Verification items for the finished model (mm, model axes). A direction names the side the tool comes from. Coordinates: 2 decimals unless noted, no trailing zeros. Write each loop counter-clockwise with the first axis right and the second up, starting at its lowest first coordinate (ties: lowest second). Pieces come first, ordered by that corner, then holes. Notation, with made-up numbers: M 73,45 L 108,45 A15 cw 108,58 Z; hole C 71.25,63 d11. An arc over 180 degrees is marked long. Answer in a Markdown table with one row per item.
from build123d import *

# Parameters (mm, degrees)
SKETCH1_W               = 80
SKETCH1_H               = 22
BOSS_EXTRUDE1_DEPTH     = 24
SKETCH2_R               = 3.85
EYESHAFT_HOLES_DEPTH    = 15
SKETCH5_W               = 5
SKETCH5_H               = 2.2
FRONT_LEG_HOLES_DEPTH   = 13
SKETCH6_W               = 20
SKETCH6_H               = 24
SERVO_BLOCK_DEPTH       = 17.5
SKETCH7_W               = 10.2
SKETCH7_H               = 3.3
BACK_LEGS_DEPTH         = 13
FILLET1_R               = 3
SKETCH8_R               = 2.714277304
CUT_EXTRUDE4_DEPTH      = 14
SKETCH9_W               = 12.2
SKETCH9_H               = 33.2
SERVO_ARMS1_DEPTH       = 11.6
FILLET2_R               = 2
CHAMFER1_SIZE           = 1
SKETCH14_W              = 12.4
SKETCH14_H              = 25
CUT_EXTRUDE5_DEPTH      = 11
SKETCH15_W              = 9
SKETCH15_H              = 4
CUT_EXTRUDE6_DEPTH      = 5.5
SKETCH16_W              = 5
SKETCH16_H              = 1
CUT_EXTRUDE7_DEPTH      = 11
SKETCH13_R              = 0.5
SERVO_SCREW_HOLES_DEPTH = 2
FILLET3_R               = 2


with BuildPart() as part:
    # Sketch1 → Boss-Extrude1 (new body)
    with BuildSketch(Plane(origin=(0, 0, 0), x_dir=(1, 0, 0), z_dir=(0, 1, 0))):
        Rectangle(SKETCH1_W, SKETCH1_H)
    extrude(amount=BOSS_EXTRUDE1_DEPTH)

    # Sketch2 → Eyeshaft holes (cut)
    with BuildSketch(Plane(origin=(0, 24, 0), x_dir=(1, 0, 0), z_dir=(0, 1, 0))):
        with Locations(Location((-30, -5, 0), (0, 0, 270))):
            Circle(SKETCH2_R)
        with Locations(Location((30, -5, 0), (0, 0, 270))):
            Circle(SKETCH2_R)
    extrude(amount=-EYESHAFT_HOLES_DEPTH, mode=Mode.SUBTRACT)

    # Sketch5 → Front leg holes (cut)
    with BuildSketch(Plane(origin=(0, 24, 0), x_dir=(1, 0, 0), z_dir=(0, 1, 0))):
        with Locations((-20, -5)):
            Rectangle(SKETCH5_W, SKETCH5_H)
        with Locations((20, -5)):
            Rectangle(SKETCH5_W, SKETCH5_H)
    extrude(amount=-FRONT_LEG_HOLES_DEPTH, mode=Mode.SUBTRACT)

    # Sketch6 → Servo block (add, symmetric)
    with BuildSketch(Plane.XY):
        with Locations((0, 12)):
            Rectangle(SKETCH6_W, SKETCH6_H)
    extrude(amount=SERVO_BLOCK_DEPTH, both=True)

    # Sketch7 → Back Legs (cut)
    with BuildSketch(Plane(origin=(0, 24, 0), x_dir=(1, 0, 0), z_dir=(0, 1, 0))):
        with Locations((-25.75, 3.4)):
            Rectangle(SKETCH7_W, SKETCH7_H)
        with Locations((25, 3.45)):
            Rectangle(SKETCH7_W, SKETCH7_H)
    extrude(amount=-BACK_LEGS_DEPTH, mode=Mode.SUBTRACT)

    # Fillet1
    fillet1_edges = [part.edges().sort_by_distance(p)[0] for p in [
        (-30, 9, 1.15),
        (30, 9, 1.15),
    ]]
    fillet(fillet1_edges, radius=FILLET1_R)

    # Sketch8 → Cut-Extrude4 (cut)
    with BuildSketch(Plane(origin=(0, 24, 0), x_dir=(1, 0, 0), z_dir=(0, 1, 0))):
        with Locations(Location((0, -5, 0), (0, 0, 270))):
            Circle(SKETCH8_R)
    extrude(amount=-CUT_EXTRUDE4_DEPTH, mode=Mode.SUBTRACT)

    # Sketch9 → Servo arms1 (cut)
    with BuildSketch(Plane(origin=(0, 24, 0), x_dir=(1, 0, 0), z_dir=(0, 1, 0))):
        Rectangle(SKETCH9_W, SKETCH9_H)
    extrude(amount=-SERVO_ARMS1_DEPTH, mode=Mode.SUBTRACT)

    # Fillet2
    fillet2_edges = [part.edges().sort_by_distance(p)[0] for p in [
        (10, 12, -11),
        (10, 12, -17.5),
        (10, 12, 11),
        (-10, 12, -11),
        (-10, 12, -17.5),
        (-10, 12, 11),
        (10, 12, 17.5),
        (-10, 12, 17.5),
        (40, 12, 11),
        (-40, 12, 11),
        (-40, 12, -11),
        (40, 12, -11),
    ]]
    fillet(fillet2_edges, radius=FILLET2_R)

    # Chamfer1
    chamfer1_edges = [part.edges().sort_by_distance(p)[0] for p in [
        (-30, 24, 1.15),
        (30, 24, 1.15),
        (-17.5, 24, 5),
        (-20, 24, 3.9),
        (-22.5, 24, 5),
        (-20, 24, 6.1),
        (22.5, 24, 5),
        (20, 24, 3.9),
        (17.5, 24, 5),
        (20, 24, 6.1),
        (-30.85, 24, -3.4),
        (-25.75, 24, -1.75),
        (-20.65, 24, -3.4),
        (-25.75, 24, -5.05),
        (19.9, 24, -3.45),
        (25, 24, -1.8),
        (30.1, 24, -3.45),
        (25, 24, -5.1),
    ]]
    chamfer(chamfer1_edges, length=CHAMFER1_SIZE)

    # Sketch14 → Cut-Extrude5 (cut)
    with BuildSketch(Plane(origin=(0, 12.4, 0), x_dir=(1, 0, 0), z_dir=(0, 1, 0))):
        with Locations((0, 0.5)):
            Rectangle(SKETCH14_W, SKETCH14_H)
    extrude(amount=-CUT_EXTRUDE5_DEPTH, mode=Mode.SUBTRACT)

    # Sketch15 → Cut-Extrude6 (cut)
    with BuildSketch(Plane.XY.offset(17.5)):
        with Locations((0, 3.4)):
            Rectangle(SKETCH15_W, SKETCH15_H)
    extrude(amount=-CUT_EXTRUDE6_DEPTH, mode=Mode.SUBTRACT)

    # Sketch16 → Cut-Extrude7 (cut)
    with BuildSketch(Plane(origin=(0, 12.4, 0), x_dir=(1, 0, 0), z_dir=(0, 1, 0))):
        with Locations((0, -12)):
            Rectangle(SKETCH16_W, SKETCH16_H)
    extrude(amount=-CUT_EXTRUDE7_DEPTH, mode=Mode.SUBTRACT)

    # Sketch13 → Servo Screw Holes (cut)
    with BuildSketch(Plane(origin=(0, 12.4, 0), x_dir=(1, 0, 0), z_dir=(0, 1, 0))):
        with Locations(Location((0.1, 15, 0), (0, 0, 270))):
            Circle(SKETCH13_R)
        with Locations(Location((0.1, -14.5, 0), (0, 0, 270))):
            Circle(SKETCH13_R)
    extrude(amount=-SERVO_SCREW_HOLES_DEPTH, mode=Mode.SUBTRACT)

    # Fillet3
    fillet3_edges = [part.edges().sort_by_distance(p)[0] for p in [
        (0, 5.4, 12.5),
        (2.5, 5.4, 12.25),
        (-2.5, 5.4, 12.25),
    ]]
    fillet(fillet3_edges, radius=FILLET3_R - 0.0001)  # a hair under: the kernel refuses the full size


solid = part.part
1) Sectioned sample at B-B (z = -4). Record the cut outline in (x, y), then the cut area to 3 significant figures.
Response values:
| item | result |
|---|---|
| outline | M -40,0 L 40,0 L 40,24 L 31.1,24 L 30.1,23 L 30.1,11 L 19.9,11 L 19.9,23 L 18.9,24 L 6.1,24 L 6.1,12.4 L 6.2,12.4 L 6.2,1.4 L -6.2,1.4 L -6.2,12.4 L -6.1,12.4 L -6.1,24 L -19.65,24 L -20.65,23 L -20.65,11 L -30.85,11 L -30.85,23 L -31.85,24 L -40,24 Z |
| area | 1,370 mm² |
2) Depth check by flat-ended pin: pin 1 (8 mm diameter, centred on x = -13.5, z = -5, fed in from -Y); pin 2 (8 mm diameter, centred on x = 27.5, y = 20, fed in from +Z); pin 3 (1.6 mm diameter, centred on x = -23.5, z = -4, fed in from +Y); pin 4 (0.8 mm diameter, centred on x = 0.5, z = -15, fed in from +Y). Enter the tip coordinate at first touch or a pass-through.
Response values:
| item | result |
|---|---|
| pin 1 | stops at y = 0 |
| pin 2 | stops at z = 11 |
| pin 3 | stops at y = 11 |
| pin 4 | stops at y = 12.4 |
3) Sectioned sample at C-C (y = 13.5). Give the number of separate pieces and of enclosed holes in the cut face, then the cut area to 3 significant figures.
Response values:
| item | result |
|---|---|
| separate pieces | 1 |
| enclosed holes | 7 |
| area | 1,430 mm² |
4) Sectioned sample at A-A (x = 21). Record the cut outline in (y, z).
Response values:
| item | result |
|---|---|
| outline | M 0,-11 L 24,-11 L 24,-6.1 L 23,-5.1 L 11,-5.1 L 11,-1.8 L 23,-1.8 L 24,-0.8 L 24,2.9 L 23,3.9 L 11,3.9 L 11,6.1 L 23,6.1 L 24,7.1 L 24,11 L 0,11 Z |
5) Sectioned sample at D-D (z = -12). Record the cut outline in (x, y).
Response values:
| item | result |
|---|---|
| outline | M -10.27,0 L 10.27,0 L 10.27,24 L 6.1,24 L 6.1,12.4 L 6.2,12.4 L 6.2,1.4 L -6.2,1.4 L -6.2,12.4 L -6.1,12.4 L -6.1,24 L -10.27,24 Z |
6) Thickness scan on L1, parallel to X at y = 20.5, z = 5; L2, parallel to X at y = 5.5, z = 4.5; L3, parallel to Z at x = 18.5, y = 15.5. Record the ranges inside material, lowest first. Write a range as [from, to].
Response values:
| item | result |
|---|---|
| L1 | x = [-40, -33.85], [-26.15, -22.5], [-17.5, -6.1], [6.1, 17.5], [22.5, 26.15], [33.85, 40] |
| L2 | x = [-40, -6.2], [6.2, 40] |
| L3 | z = [-11, 3.9], [6.1, 11] |
7) Tool access check on faces 1 (the face through (-10, 12, -14)), 2 (the face through (-20.65, 17, -3)), 3 (the face through (-4.5, 3, 15)), 4 (the face through (-10, 12, 14)). Record the directions out of +Z, -Z, +X, -X, +Y, -Y that give a thin tool (end or side, any length) a straight path to the whole face; none if there is none.
Response values:
| item | result |
|---|---|
| face 1 | -Z, -X, +Y, -Y |
| face 2 | +Y |
| face 3 | +Z |
| face 4 | +Z, -X, +Y, -Y |
8) Release check for a two-part mould opening along X. For faces 5 (the face through (-9.43, 12.17, 16.9)), 6 (the face through (-30.85, 17, -3)), 7 (the face through (25, 12, 11)), 8 (the face through (10, 12, -14)) record: +X half, -X half, draft (parallel to the pull), parting line (faces both ways), or undercut.
Response values:
| item | result |
|---|---|
| face 5 | -X half |
| face 6 | undercut |
| face 7 | draft |
| face 8 | +X half |
